```python
from build123d import *

# Parameters (mm, degrees)
F0_W      = 104.7
F0_H      = 44.2
F0_W_2    = 98.7
F0_H_2    = 38.2
F1_DEPTH  = 90
F2_W      = 98.7
F2_H      = 38.2
F3_DEPTH  = 3
F4_R      = 1.5
F5_DEPTH  = 3
F6_R      = 3
F7_DEPTH  = 1
F8_W      = 48.4
F8_H      = 28
F8_R      = 1.75
F9_DEPTH  = 3
F10_SIZE  = 5
F11_W     = 8
F11_H     = 20
F12_DEPTH = 3
F13_SIZE  = 1
F14_SIZE  = 1
F15_SIZE  = 0.5


with BuildPart() as f1:
    # F0 (on Top) → F1 (new body)
    with BuildSketch(Plane.XY):
        Rectangle(F0_W, F0_H)
        Rectangle(F0_W_2, F0_H_2, mode=Mode.SUBTRACT)
    extrude(amount=F1_DEPTH)

    # F2 (on face) → F3 (join)
    with BuildSketch(Plane(origin=(0, 0, 0), x_dir=(1, 0, 0), z_dir=(0, 0, -1))):
        Rectangle(F2_W, F2_H)
    extrude(amount=-F3_DEPTH)

    # F4 (on face) → F5 (cut)
    with BuildSketch(Plane(origin=(49.35, 0, 0), x_dir=(0, -1, 0), z_dir=(-1, 0, 0))):
        with Locations((1.1, 80)):
            Circle(F4_R)
    extrude(amount=-F5_DEPTH, mode=Mode.SUBTRACT)

    # F6 (on face) → F7 (cut)
    with BuildSketch(Plane.YZ.offset(52.35)):
        with Locations((-1.1, 80)):
            Circle(F6_R)
    extrude(amount=-F7_DEPTH, mode=Mode.SUBTRACT)

    # F8 (on face) → F9 (cut)
    with BuildSketch(Plane(origin=(0, 22.1, 0), x_dir=(-1, 0, 0), z_dir=(0, 1, 0))):
        with Locations((19.15, 28)):
            Rectangle(F8_W, F8_H)
        with Locations((19.15, 8)):
            Circle(F8_R)
        with Locations((19.15, 48)):
            Circle(F8_R)
    extrude(amount=-F9_DEPTH, mode=Mode.SUBTRACT)

    # F10
    f10_edges = [f1.edges().sort_by_distance(p)[0] for p in [
        (-43.35, 20.6, 42),
        (-43.35, 20.6, 14),
    ]]
    chamfer(f10_edges, length=F10_SIZE)

    # F11 (on face) → F12 (cut)
    with BuildSketch(Plane(origin=(0, 22.1, 0), x_dir=(-1, 0, 0), z_dir=(0, 1, 0))):
        with Locations((-44.35, 14)):
            Rectangle(F11_W, F11_H)
        with Locations((-44.35, 39)):
            Rectangle(F11_W, F11_H)
    extrude(amount=-F12_DEPTH, mode=Mode.SUBTRACT)

    # F13
    f13_edges = [f1.edges().sort_by_distance(p)[0] for p in [
        (40.35, 20.6, 24),
        (48.35, 20.6, 24),
        (48.35, 20.6, 4),
        (40.35, 20.6, 4),
        (48.35, 20.6, 29),
        (40.35, 20.6, 29),
        (40.35, 20.6, 49),
        (48.35, 20.6, 49),
    ]]
    chamfer(f13_edges, length=F13_SIZE)

    # F14
    f14_edges = [f1.edges().sort_by_distance(p)[0] for p in [
        (0, 22.1, 0),
        (-52.35, 0, 0),
        (0, -22.1, 0),
        (52.35, 0, 0),
        (52.35, 22.1, 45),
        (52.35, -22.1, 45),
        (-52.35, -22.1, 45),
        (-52.35, 22.1, 45),
    ]]
    chamfer(f14_edges, length=F14_SIZE)

    # F15
    f15_edges = [f1.edges().sort_by_distance(p)[0] for p in [
        (0, -19.1, 3),
        (-49.35, 0, 3),
        (0, 19.1, 3),
        (49.35, 0, 3),
    ]]
    chamfer(f15_edges, length=F15_SIZE)


solid = f1.part
```
The listing builds one solid part. Answer for the finished solid, in the listing's coordinates (mm). A direction names the side the tool comes from. Give positions to 0.01 mm unless a question says otherwise; leave off trailing zeros. Write each loop counter-clockwise with the first axis right and the second up, starting at its lowest first coordinate (ties: lowest second). Pieces come first, ordered by that corner, then holes. Notation, with made-up numbers: (42.25, -15.75) - (76.25, -15.75) arc R22 cw to (76.25, 18.25) - close; hole circle Ø5 at (40.5, 26). An arc over 180 degrees is marked (long way). Use one line per item in the form item = value. Start each with the question number.
1) Find section D-D on y = -1.1. Determine the outline of the cut face in (x, z).
2) Find section A-A on x = -33.5. Determine the outline of the cut face in (y, z), plus the area to 3 significant figures.
3) Flat-ended cylindrical pins translate along their axes: pin 1 Ø5 at (y, z) = (-1.1, 80) entering from +X; pin 2 Ø4 at (x, y) = (6.5, 4.5) entering from +Z; pin 3 Ø2 at (x, z) = (-19.15, 8) entering from +Y. Find the tip coordinate at first contact, or state that the pin passes through.
4) Find section B-B on z = 8. Determine the outline of the cut face in (x, y), plus the area to 3 significant figures.
5) The mould has two halves that part along X. Classify faces 1 (the face through (49.35, 0, 46)), 2 (the face through (-1, -22.1, 45)), 3 (the face through (52.35, 0, 45)): pulls with the +X half, pulls with the -X half, needs draft (parallel to the pull), parting line crosses it, or undercut.
6) Consider line 1 along Z through (x, y) = (-19.15, 20.4); line 2 along Y through (x, z) = (-45.5, 15); line 3 along X through (y, z) = (-19, 39). Determine where each line is inside the solid, lowest interval first. Write a range as from..to.
7) Find section C-C on x = -19.15. Determine the outline of the cut face in (y, z).
8) A tool of negligible diameter and unlimited length cuts with its end or side. For faces 4 (the face through (51.86, -1.75, 77.07)), 5 (the face through (44, 21, 29)), 6 (the face through (-1, 0, 3)), from which of +Z, -Z, +X, -X, +Y, -Y can it reach the whole face along a straight path? Write none if from no direction.
Geometry results:
q1.outline = (-52.35, 1) - (-51.35, 0) - (51.35, 0) - (52.35, 1) - (52.35, 77) - (51.35, 77) - (51.35, 78.5) - (49.35, 78.5) - (49.35, 3.5) - (48.85, 3) - (-48.85, 3) - (-49.35, 3.5) - (-49.35, 90) - (-52.35, 90) - close; (49.35, 81.5) - (51.35, 81.5) - (51.35, 83) - (52.35, 83) - (52.35, 90) - (49.35, 90) - close
q2.outline = (-22.1, 1) - (-21.1, 0) - (21.1, 0) - (22.1, 1) - (22.1, 14) - (19.1, 14) - (19.1, 3.5) - (18.6, 3) - (-18.6, 3) - (-19.1, 3.5) - (-19.1, 90) - (-22.1, 90) - close; (19.1, 42) - (22.1, 42) - (22.1, 90) - (19.1, 90) - close
q2.area = 570 mm2
q3.pin_1 = 51.35
q3.pin_2 = 3
q3.pin_3 = -19.1
q4.outline = (-52.35, -21.1) - (-51.35, -22.1) - (51.35, -22.1) - (52.35, -21.1) - (52.35, 21.1) - (51.35, 22.1) - (48.35, 22.1) - (48.35, 19.1) - (49.35, 19.1) - (49.35, -19.1) - (-49.35, -19.1) - (-49.35, 19.1) - (-20.9, 19.1) - (-20.9, 22.1) - (-51.35, 22.1) - (-52.35, 21.1) - close; (-17.4, 19.1) - (40.35, 19.1) - (40.35, 22.1) - (-17.4, 22.1) - close
q4.area = 821 mm2
q5.face_1 = undercut
q5.face_2 = needs draft
q5.face_3 = pulls with the +X half
q6.line_1 = 0..6.25, 9.75..14, 42..46.25, 49.75..90
q6.line_2 = -22.1..-19.1, 19.1..22.1
q6.line_3 = -52.35..-49.35, 49.35..52.35
q7.outline = (-22.1, 1) - (-21.1, 0) - (21.1, 0) - (22.1, 1) - (22.1, 6.25) - (19.1, 6.25) - (19.1, 3.5) - (18.6, 3) - (-18.6, 3) - (-19.1, 3.5) - (-19.1, 90) - (-22.1, 90) - close; (19.1, 9.75) - (22.1, 9.75) - (22.1, 14) - (19.1, 14) - close; (19.1, 42) - (22.1, 42) - (22.1, 46.25) - (19.1, 46.25) - close; (19.1, 49.75) - (22.1, 49.75) - (22.1, 90) - (19.1, 90) - close
q8.face_4 = +X
q8.face_5 = +Y
q8.face_6 = +Z
